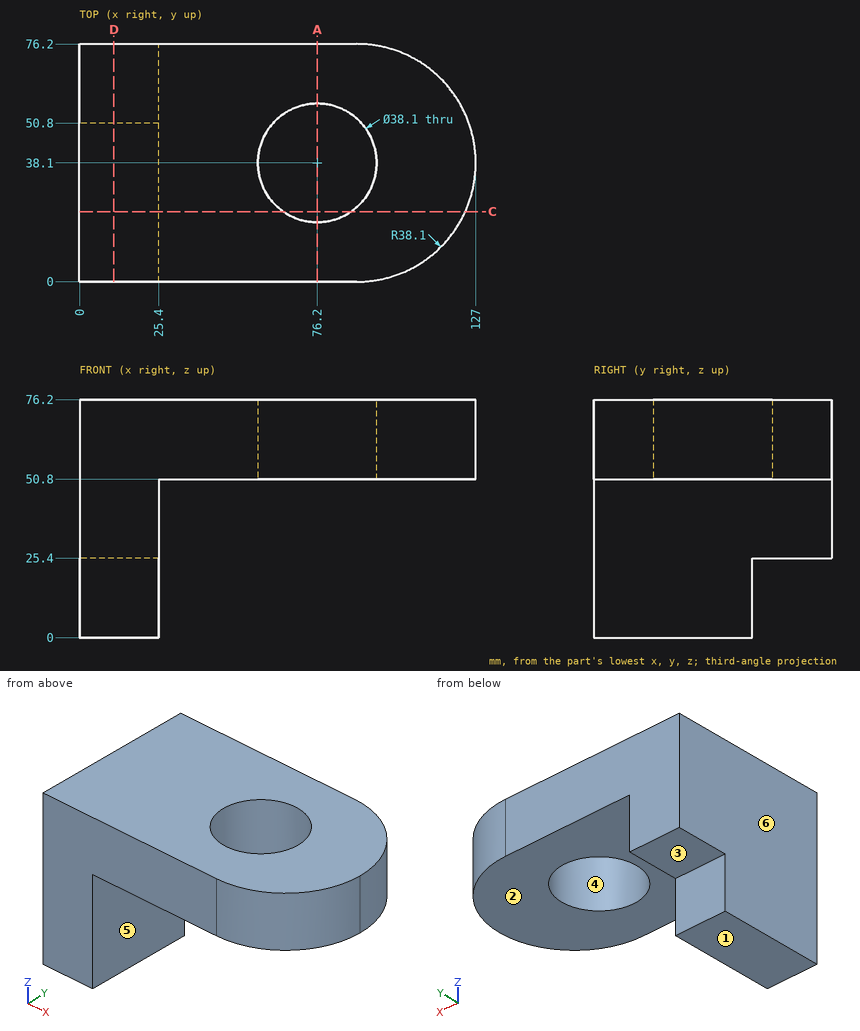
Job drawing, mm, ordinate dimensions from the low corner. One solid piece. A direction names the side the tool comes from. Give positions to 0.01 mm unless a question says otherwise; leave off trailing zeros. Order: outer loops, then holes, each group sorted by start corner. A loop starts at its lowest first (then second) coordinate and runs counter-clockwise, first axis right, second up. Notation, with made-up numbers: M 64,-28.5 L 77,-28.5 A15 ccw 77,-13.5 Z; hole C 38.25,-35.5 d2. An arc over 180 degrees is marked long. Put each result on its own line as item: value. Start each with the question number.
(1) Tool access for the marked faces 1, 2 and 3: list every direction of +Z, -Z, +X, -X, +Y, -Y with a clear straight run to the whole face (end or side of a thin tool).
(2) Drill centre lines: L1, parallel to X at y = 38, z = 59; L2, parallel to Y at x = 76.2, z = 66.25; L3, parallel to Z at x = 49.5, y = 62. Where is each one in solid material? Low to high. Write a range as [from, to].
(3) Pin check, flat tips, straight feed: pin 1 Ø6 at (x, z) = (91.5, 61.5) entering from +Y; pin 2 Ø12 at (y, z) = (15, 59) entering from +X; pin 3 Ø1.5 at (y, z) = (14.5, 45) entering from +X. Stop position of each tip, or through.
(4) Band-saw the part on A-A on x = 76.2. Give the cut face in (y, z), then the cut area to 3 significant figures.
(5) Band-saw the part on D-D on x = 11. Give the cut face in (y, z).
(6) Pull direction X, two halves, no side cores. Call the marked faces 4, 5 and 6: released by +X, released by -X, zero draft, split by the parting line, or undercut.
(7) Band-saw the part on C-C on y = 22.5. Give the cut face in (x, z).
Results below:
1. face 1: -Z, +X, -X, +Y, -Y
1. face 2: -Z, +X, +Y, -Y
1. face 3: -Z, +X, -X, +Y
2. L1: x = [0, 57.15], [95.25, 127]
2. L2: y = [0, 19.05], [57.15, 76.2]
2. L3: z = [50.8, 76.2]
3. pin 1: stops at y = 76.2
3. pin 2: stops at x = 122.95
3. pin 3: stops at x = 25.4
4. outline: M 0,50.8 L 19.05,50.8 L 19.05,76.2 L 0,76.2 Z; M 57.15,50.8 L 76.2,50.8 L 76.2,76.2 L 57.15,76.2 Z
4. area: 968 mm2
5. outline: M 0,0 L 50.8,0 L 50.8,25.4 L 76.2,25.4 L 76.2,76.2 L 0,76.2 Z
6. face 4: undercut
6. face 5: released by +X
6. face 6: released by -X
7. outline: M 0,0 L 25.4,0 L 25.4,50.8 L 65.27,50.8 L 65.27,76.2 L 0,76.2 Z; M 87.13,50.8 L 123.66,50.8 L 123.66,76.2 L 87.13,76.2 Z
